Can you work these out from the model? Positions are in its coordinate system, mm. Face numbers are marked on the shaded views. Give positions to 0.01 mm unless a question says otherwise; leave off trailing zeros. Order: outer loops, then holes, each group sorted by start corner. A loop starts at its lowest first (then second) coordinate and runs counter-clockwise, first axis right, second up. Notation, with made-up numbers: M 61.5,46 L 109.5,46 A24 cw 109.5,61 Z; hole C -5.75,19 d8. An arc over 180 degrees is marked long. Use one line per item in the form item = value. Start each with the question number.
1. I want a section at B-B, the plane z = -16. List the corners of the cut face in (x, y) for me, and give its area (3 significant figures).
2. We'd pull the mould along Z, two halves only. Please class the marked faces 1, 2 and 3: +Z half, -Z half, draft (parallel to the pull), parting line (faces both ways), or undercut.
3. I want a section at D-D, the plane x = 2.25. Count the separate pieces of the cut face and the enclosed holes in it, and give its area (3 significant figures).
4. I want a section at C-C, the plane y = 39. List the corners of the cut face in (x, z) for me, and give its area (3 significant figures).
5. I want a section at A-A, the plane y = 60. List the corners of the cut face in (x, z) for me, and give its area (3 significant figures).
6. I need wall thicknesses on L1, parallel to Y at x = 2.8, z = -20.5 (3 decimals); L2, parallel to Y at x = 1.75, z = -32; L3, parallel to Y at x = 1.2, z = -20. Which ranges of each line are inside material? Lowest first, please.
7. Will these pins go through, and if not, where does the flat tip stop? P1, Ø1.5, axis at x = 4, y = 33, coming from the +Z side; P2, Ø5, axis at y = 24, z = -32, coming from the +X side; P3, Ø2.5, axis at y = 12, z = -8, coming from the +X side.
```python
from build123d import *

# Parameters (mm, degrees)
CROQUIS1_R              = 2
CROQUIS1_R_2            = 2.5
CROQUIS1_R_3            = 11
SALIENTE_EXTRUIR1_DEPTH = 5


with BuildPart() as part:
    # Croquis1 → Saliente-Extruir1 (new body)
    with BuildSketch(Plane(origin=(0, 0, 0), x_dir=(0, 0, -1), z_dir=(1, 0, 0))):
        with BuildLine():
            ThreePointArc((43.892972847, 52.642972847), (20, 85), (-3.892972847, 52.642972847))
            Line((-3.892972847, 52.642972847), (0, 40))
            Line((0, 40), (0, 0))
            Line((0, 0), (40, 0))
            Line((40, 0), (40, 40))
            Line((40, 40), (43.892972847, 52.642972847))
        make_face()
        with Locations((8, 12)):
            Circle(CROQUIS1_R, mode=Mode.SUBTRACT)
        with Locations((8, 24)):
            Circle(CROQUIS1_R, mode=Mode.SUBTRACT)
        with Locations((20, 39)):
            Circle(CROQUIS1_R_2, mode=Mode.SUBTRACT)
        with Locations((32, 12)):
            Circle(CROQUIS1_R, mode=Mode.SUBTRACT)
        with Locations((32, 24)):
            Circle(CROQUIS1_R, mode=Mode.SUBTRACT)
        with Locations((-1, 60)):
            Circle(CROQUIS1_R_2, mode=Mode.SUBTRACT)
        with Locations((20, 60)):
            Circle(CROQUIS1_R_3, mode=Mode.SUBTRACT)
        with Locations((20, 81)):
            Circle(CROQUIS1_R_2, mode=Mode.SUBTRACT)
        with Locations((41, 60)):
            Circle(CROQUIS1_R_2, mode=Mode.SUBTRACT)
    extrude(amount=SALIENTE_EXTRUIR1_DEPTH)


solid = part.part
```
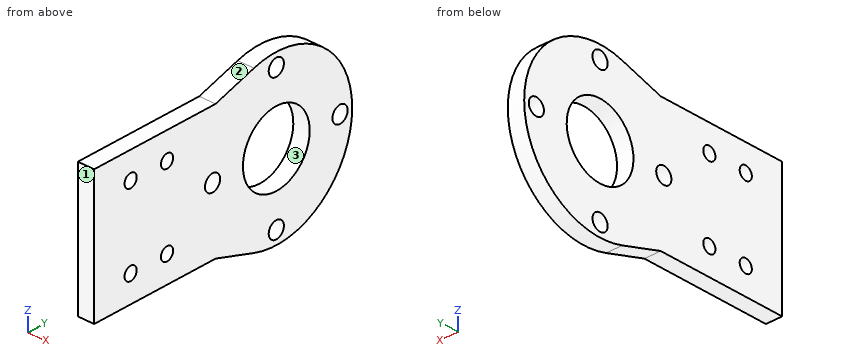
Check result:
q1.outline = M 0,0 L 5,0 L 5,49.75 L 0,49.75 Z; M 0,70.25 L 5,70.25 L 5,84.68 L 0,84.68 Z
q1.area = 321 mm2
q2.face_1 = draft
q2.face_2 = +Z half
q2.face_3 = undercut
q3.separate_pieces = 1
q3.enclosed_holes = 9
q3.area = 2,990 mm2
q4.outline = M 0,-40 L 5,-40 L 5,-22.5 L 0,-22.5 Z; M 0,-17.5 L 5,-17.5 L 5,0 L 0,0 Z
q4.area = 175 mm2
q5.outline = M 0,-45 L 5,-45 L 5,-43.5 L 0,-43.5 Z; M 0,-38.5 L 5,-38.5 L 5,-31 L 0,-31 Z; M 0,-9 L 5,-9 L 5,-1.5 L 0,-1.5 Z; M 0,3.5 L 5,3.5 L 5,5 L 0,5 Z
q5.area = 90.0 mm2
q6.L1 = 0 to 36.551, 41.449 to 49.011, 70.989 to 78.551, 83.449 to 84.995
q6.L2 = 0 to 10, 14 to 22, 26 to 81.93
q6.L3 = 0 to 36.5, 41.5 to 49, 71 to 78.5, 83.5 to 85
q7.P1 = 0
q7.P2 = 5
q7.P3 = through
